from build123d import *

# Parameters (mm, degrees)
F0_R     = 4
F0_R_2   = 3
F0_R_3   = 3.25
F1_DEPTH = 6
F3_DEPTH = 12.5
F5_DEPTH = 1.25
F6_W     = 9.5
F6_H     = 2
F7_DEPTH = 25
F9_DEPTH = 2


with BuildPart() as f1:
    # F0 (on Front) → F1 (new body)
    with BuildSketch(Plane.XZ):
        with BuildLine():
            ThreePointArc((-13, 5), (-9.4644660941, 3.5355339059), (-8, 0))
            ThreePointArc((-8, 0), (-9.4644660941, -3.5355339059), (-13, -5))
            Line((-13, -5), (13, -5))
            ThreePointArc((13, -5), (8, 0), (13, 5))
            Line((13, 5), (9, 5))
            ThreePointArc((9, 5), (6.1715728753, 6.1715728753), (5, 9))
            Line((5, 9), (5, 23.5))
            ThreePointArc((5, 23.5), (0, 28.5), (-5, 23.5))
            Line((-5, 23.5), (-5, 9))
            ThreePointArc((-5, 9), (-6.1715728753, 6.1715728753), (-9, 5))
            Line((-9, 5), (-13, 5))
        make_face()
        Circle(F0_R, mode=Mode.SUBTRACT)
        with Locations((0, 23.5)):
            Circle(F0_R_2, mode=Mode.SUBTRACT)
        with BuildLine():
            ThreePointArc((-13, -5), (-9.4644660941, -3.5355339059), (-8, 0))
            ThreePointArc((-8, 0), (-9.4644660941, 3.5355339059), (-13, 5))
            ThreePointArc((-13, 5), (-18, 0), (-13, -5))
        make_face()
        with Locations((-13, 0)):
            Circle(F0_R_3, mode=Mode.SUBTRACT)
        with BuildLine():
            ThreePointArc((13, 5), (8, 0), (13, -5))
            ThreePointArc((13, -5), (16.5355339059, -3.5355339059), (18, 0))
            ThreePointArc((18, 0), (16.5355339059, 3.5355339059), (13, 5))
        make_face()
        with Locations((13, 0)):
            Circle(F0_R_3, mode=Mode.SUBTRACT)
    extrude(amount=F1_DEPTH)

    # F2 (on Right) → F3 (cut, symmetric)
    with BuildSketch(Plane.YZ):
        with BuildLine():
            Line((0, 28.5), (-4, 28.5))
            Line((-4, 28.5), (-4, 12.0710678119))
            ThreePointArc((-4, 12.0710678119), (-3.6193976626, 10.15765065), (-2.5355339059, 8.5355339059))
            Line((-2.5355339059, 8.5355339059), (0, 6))
            Line((0, 6), (0, 28.5))
        make_face()
    extrude(amount=F3_DEPTH, both=True, mode=Mode.SUBTRACT)

    # F4 (on Right) → F5 (join, symmetric)
    with BuildSketch(Plane.YZ):
        with BuildLine():
            Line((-2.5355339059, 8.5355339059), (0, 6))
            Line((0, 6), (-4, 19.0834104739))
            Line((-4, 19.0834104739), (-4, 12.0710678119))
            ThreePointArc((-4, 12.0710678119), (-3.6193976626, 10.15765065), (-2.5355339059, 8.5355339059))
        make_face()
    extrude(amount=F5_DEPTH, both=True)

    # F6 (on face) → F7 (cut)
    with BuildSketch(Plane.XY.offset(5)):
        with Locations((13.25, -3)):
            Rectangle(F6_W, F6_H)
        with Locations((-13.25, -3)):
            Rectangle(F6_W, F6_H)
    extrude(amount=-F7_DEPTH, mode=Mode.SUBTRACT)

    # F8 (on face) → F9 (cut)
    with BuildSketch(Plane(origin=(0, 0, 0), x_dir=(-1, 0, 0), z_dir=(0, 1, 0))):
        with BuildLine():
            Line((13.75, 6.816144567), (12.25, 6.816144567))
            Line((12.25, 6.816144567), (12.25, 3.1622776602))
            ThreePointArc((12.25, 3.1622776602), (13, 3.25), (13.75, 3.1622776602))
            Line((13.75, 3.1622776602), (13.75, 6.816144567))
        make_face()
        with BuildLine():
            ThreePointArc((13.75, 3.1622776602), (13, 3.25), (12.25, 3.1622776602))
            Line((12.25, 3.1622776602), (12.25, 1.0694904486))
            Line((12.25, 1.0694904486), (13.75, 1.0694904486))
            Line((13.75, 1.0694904486), (13.75, 3.1622776602))
        make_face()
        with BuildLine():
            Line((12.25, 1.0694904486), (12.25, 3.1622776602))
            ThreePointArc((12.25, 3.1622776602), (10.9844355629, -2.5495097568), (16.25, 0))
            ThreePointArc((16.25, 0), (15.5495097568, 2.0155644371), (13.75, 3.1622776602))
            Line((13.75, 3.1622776602), (13.75, 1.0694904486))
            Line((13.75, 1.0694904486), (12.25, 1.0694904486))
        make_face()
        with BuildLine():
            ThreePointArc((-13.75, 3.1622776602), (-15.0155644371, -2.5495097568), (-9.75, 0))
            ThreePointArc((-9.75, 0), (-10.4504902432, 2.0155644371), (-12.25, 3.1622776602))
            Line((-12.25, 3.1622776602), (-12.25, 1.0694904486))
            Line((-12.25, 1.0694904486), (-13.75, 1.0694904486))
            Line((-13.75, 1.0694904486), (-13.75, 3.1622776602))
        make_face()
        with BuildLine():
            Line((-12.25, 1.0694904486), (-12.25, 3.1622776602))
            ThreePointArc((-12.25, 3.1622776602), (-13, 3.25), (-13.75, 3.1622776602))
            Line((-13.75, 3.1622776602), (-13.75, 1.0694904486))
            Line((-13.75, 1.0694904486), (-12.25, 1.0694904486))
        make_face()
        with BuildLine():
            ThreePointArc((-13.75, 3.1622776602), (-13, 3.25), (-12.25, 3.1622776602))
            Line((-12.25, 3.1622776602), (-12.25, 6.816144567))
            Line((-12.25, 6.816144567), (-13.75, 6.816144567))
            Line((-13.75, 6.816144567), (-13.75, 3.1622776602))
        make_face()
        with BuildLine():
            ThreePointArc((-12.25, 3.1622776602), (-13, 3.25), (-13.75, 3.1622776602))
            Line((-13.75, 3.1622776602), (-13.75, 1.0694904486))
            Line((-13.75, 1.0694904486), (-12.25, 1.0694904486))
            Line((-12.25, 1.0694904486), (-12.25, 3.1622776602))
        make_face()
        with BuildLine():
            Line((-13.75, 1.0694904486), (-13.75, 3.1622776602))
            ThreePointArc((-13.75, 3.1622776602), (-15.0155644371, -2.5495097568), (-9.75, 0))
            ThreePointArc((-9.75, 0), (-10.4504902432, 2.0155644371), (-12.25, 3.1622776602))
            Line((-12.25, 3.1622776602), (-12.25, 1.0694904486))
            Line((-12.25, 1.0694904486), (-13.75, 1.0694904486))
        make_face()
    extrude(amount=-F9_DEPTH, mode=Mode.SUBTRACT)


solid = f1.part
Here's how the part is built. I have some questions about the finished solid (model axes, mm). A direction names the side the tool comes from. Give positions to 0.01 mm unless a question says otherwise; leave off trailing zeros. Order: outer loops, then holes, each group sorted by start corner. A loop starts at its lowest first (then second) coordinate and runs counter-clockwise, first axis right, second up. Notation, with made-up numbers: (74.5, 78.25) -> (122.5, 78.25) arc R23 cw to (122.5, 109.25) -> close; hole circle Ø8 at (-20, -31.75). An arc over 180 degrees is marked (long way). Use a Markdown table: item, result. Add a question column.
Item 1: Will these pins go through, and if not, where does the flat tip stop? pin 1 (12 mm diameter, centred on x = 0, z = 1, fed in from +Y); pin 2 (2 mm diameter, centred on x = -10, y = -0.5, fed in from +Z); pin 3 (1 mm diameter, centred on y = -3, z = -1, fed in from -X); pin 4 (2 mm diameter, centred on y = -1.5, z = 13.5, fed in from -X).
Item 2: I need wall thicknesses on line 1 (Z direction, x = 0, y = -5.25); line 2 (Z direction, x = 13, y = -4.9); line 3 (X direction, y = -4.4, z = 23.5). Which ranges of each line are inside material? Lowest first, please.
Item 3: Imagine slicing it at D-D on z = 21. Please give me the cut outline in (x, y), plus the area to 3 significant figures.
Item 4: If we mould it in two halves opening along X, with no side actions, what happens to faces 5 (the face through (9.753, -4.986, 0.143)), 6 (the face through (-3, -1, 7)), 7 (the face through (-6.141, -2.958, 6.203))? For each: pulls with the +X half, pulls with the -X half, needs draft (parallel to the pull), parting line crosses it, or undercut.
Item 5: Imagine slicing it at A-A on x = 0. Please give me the cut outline in (y, z).
Item 6: For faces 1 (the face through (12.1, -2, -3.3)), 2 (the face through (-3.11, -3.63, 10.18)), 3 (the face through (3, -1, 7)), 4 (the face through (13.75, -1, 4)), which set-ups out of +Z, -Z, +X, -X, +Y, -Y let a thin tool reach every point of the face, with its end or its side?
Item 7: Imagine slicing it at B-B on x = 10.5. Please give me the cut outline in (y, z).
Item 8: Imagine slicing it at C-C on y = -5. Please give me the cut outline in (x, z), plus the area to 3 significant figures.
Data:
| question | item | result |
|---|---|---|
| 1 | pin 1 | stops at y = 0 |
| 1 | pin 2 | stops at z = 5 |
| 1 | pin 3 | stops at x = -8.5 |
| 1 | pin 4 | stops at x = -1.25 |
| 2 | line 1 | z = -5 to -4, 4 to 20.5, 26.5 to 28.5 |
| 2 | line 2 | z = -5 to -3.25, 3.25 to 5 |
| 2 | line 3 | x = -5 to -3, 3 to 5 |
| 3 | outline | (-5, -6) -> (-1.66, -6) -> (-1.66, -4) -> (-5, -4) -> close; (1.66, -6) -> (5, -6) -> (5, -4) -> (1.66, -4) -> close |
| 3 | area | 13.4 mm² |
| 4 | face 5 | undercut |
| 4 | face 6 | needs draft |
| 4 | face 7 | pulls with the -X half |
| 5 | outline | (-6, -5) -> (0, -5) -> (0, -4) -> (-6, -4) -> close; (-6, 4) -> (0, 4) -> (0, 6) -> (-4, 19.08) -> (-4, 20.5) -> (-6, 20.5) -> close; (-6, 26.5) -> (-4, 26.5) -> (-4, 28.5) -> (-6, 28.5) -> close |
| 6 | face 1 | -Z, +X |
| 6 | face 2 | +Z, -X, +Y |
| 6 | face 3 | +Z, +X, +Y |
| 6 | face 4 | +Z, +Y |
| 7 | outline | (-6, -5) -> (-4, -5) -> (-4, -2.08) -> (-6, -2.08) -> close; (-6, 2.08) -> (-4, 2.08) -> (-4, 5) -> (-6, 5) -> close; (-2, -5) -> (0, -5) -> (0, -2.08) -> (-2, -2.08) -> close; (-2, 2.08) -> (0, 2.08) -> (0, 5) -> (-2, 5) -> close |
| 8 | outline | (-13, -5) -> (13, -5) arc R5 ccw to (13, 5) -> (9, 5) arc R4 cw to (5, 9) -> (5, 23.5) arc R5 ccw to (-5, 23.5) -> (-5, 9) arc R4 cw to (-9, 5) -> (-13, 5) arc R5 ccw to start; hole circle Ø6.5 at (-13, 0); hole circle Ø8 at (0, 0); hole circle Ø6 at (0, 23.5); hole circle Ø6.5 at (13, 0) |
| 8 | area | 425 mm² |
